from build123d import *

# Parameters (mm, degrees)
BOSS_EXTRUDE1_DEPTH     = 20
SKETCH3_R               = 1.632108338
CUT_EXTRUDE1_DEPTH      = 33.330326321
CUT_EXTRUDE1_DEPTH_BACK = 33.330326321
SKETCH4_W               = 30
SKETCH4_H               = 41
BOSS_EXTRUDE2_DEPTH     = 5
SKETCH6_W               = 25
SKETCH6_H               = 25
BOSS_EXTRUDE3_DEPTH     = 20
CUT_EXTRUDE4_START      = 12.5
CUT_EXTRUDE4_DEPTH      = 20
SKETCH8_W               = 9.9
SKETCH8_H               = 9.9
SKETCH8_W_2             = 15.1
CUT_EXTRUDE5_DEPTH      = 33.330326321
CUT_EXTRUDE5_DEPTH_BACK = 33.330326321


with BuildPart() as part:
    # Sketch2 → Boss-Extrude1 (new body)
    with BuildSketch(Plane.XY):
        Polygon((0, 20.5), (-15, 20.5), (-15, 6.5), (-5.864885696, 6.5), (-5.864885696, -6.5), (-15, -6.5), (-15, -20.5), (0, -20.5), (15, -20.5), (15, -6.5), (5.864885696, -6.5), (5.864885696, 6.5), (15, 6.5), (15, 20.5), align=None)
    extrude(amount=BOSS_EXTRUDE1_DEPTH)

    # Sketch3 → Cut-Extrude1 (cut, two sides)
    with BuildSketch(Plane(origin=(0, 0, 0), x_dir=(1, 0, 0), z_dir=(0, 1, 0))) as cut_extrude1_sk:
        with Locations(Location((-10, -10, 0), (0, 0, 270))):
            Circle(SKETCH3_R)
        with Locations(Location((10, -10, 0), (0, 0, 270))):
            Circle(SKETCH3_R)
    extrude(amount=CUT_EXTRUDE1_DEPTH, mode=Mode.SUBTRACT)
    extrude(cut_extrude1_sk.sketch, amount=-CUT_EXTRUDE1_DEPTH_BACK, mode=Mode.SUBTRACT)

    # Sketch4 → Boss-Extrude2 (add)
    with BuildSketch(Plane.XY):
        Rectangle(SKETCH4_W, SKETCH4_H)
    extrude(amount=BOSS_EXTRUDE2_DEPTH)

    # Sketch6 → Boss-Extrude3 (add)
    with BuildSketch(Plane.XY):
        Rectangle(SKETCH6_W, SKETCH6_H)
    extrude(amount=-BOSS_EXTRUDE3_DEPTH)

    # Sketch7 → Cut-Extrude4 (cut)
    with BuildSketch(Plane(origin=(0, 0, 0), x_dir=(1, 0, 0), z_dir=(0, 1, 0)).offset(CUT_EXTRUDE4_START)):
        Polygon((-2.6, 5.15), (-7.55, 5.15), (-7.55, 0), (0, 0), (0, 10.1), (-2.6, 10.1), align=None)
        Polygon((0, 10.1), (0, 0), (7.55, 0), (7.55, 5.15), (2.6, 5.15), (2.6, 10.1), align=None)
    extrude(amount=-CUT_EXTRUDE4_DEPTH, mode=Mode.SUBTRACT)

    # Sketch8 → Cut-Extrude5 (cut, two sides)
    with BuildSketch(Plane(origin=(0, 0, 0), x_dir=(1, 0, 0), z_dir=(0, 1, 0))) as cut_extrude5_sk:
        with Locations((-7.55, 15.05)):
            Rectangle(SKETCH8_W, SKETCH8_H)
        with Locations((4.95, 15.05)):
            Rectangle(SKETCH8_W_2, SKETCH8_H)
    extrude(amount=CUT_EXTRUDE5_DEPTH, mode=Mode.SUBTRACT)
    extrude(cut_extrude5_sk.sketch, amount=-CUT_EXTRUDE5_DEPTH_BACK, mode=Mode.SUBTRACT)


solid = part.part
Can you work these out from the model? Positions are in its coordinate system, mm. A direction names the side the tool comes from. Coordinates: 2 decimals unless noted, no trailing zeros. Loops run counter-clockwise (first coordinate to the right, second up) from the corner with the lowest first, then second, coordinate; pieces in that order, holes last. Notation, with made-up numbers: (11, 12) - (62, 12) arc R19 cw to (62, 19) - close; hole circle Ø7 at (41, -3). An arc over 180 degrees is marked (long way). Answer as a JSON object with one key per item and string values. Group by question number.
Item 1: If we section it at B-B (x = -10): List the corners of the cut face in (y, z) for me.
Item 2: For pin 1 (5.5 mm diameter, centred on y = 7, z = -6.5, fed in from -X); pin 2 (2.5 mm diameter, centred on x = 9.5, y = -2, fed in from +Z); pin 3 (12 mm diameter, centred on x = 2, z = -6.5, fed in from +Y), each with a flat end and sliding along its axis, tell me the tip position at first contact or that it passes through.
Item 3: If we section it at A-A (z = 10): List the corners of the cut face in (x, y) for me, plus the area to 3 significant figures.
Item 4: If I drill on L1, parallel to X at y = 17, z = 10; L2, parallel to Z at x = -10, y = 10.5; L3, parallel to Z at x = -7.25, y = 3.5, over which ranges is the centre line in solid material (lowest first)? Write a range as from..to.
Item 5: On a 3-axis mill with a long thin cutter (end or side, diameter ignored), from which of +Z, -Z, +X, -X, +Y, -Y can I reach the whole of each face in a straight line? I mean faces 1 (the face through (-2.6, 3, -8)), 2 (the face through (0, -12.5, -5)), 3 (the face through (10, 0, 5)), 4 (the face through (-5, 3, -5.15)). Say none if no direction works.
Item 6: If we section it at D-D (x = -4.5): List the corners of the cut face in (y, z) for me, plus the area to 4 significant figures.
Item 7: If we section it at C-C (y = -13.5): List the corners of the cut face in (x, z) for me.
Item 8: If we mould it in two halves opening along Y, with no side actions, what happens to faces 5 (the face through (-12.5, 0, -5)), 6 (the face through (-9, 12.5, -6)), 7 (the face through (-10, 6.5, 12))? For each: released by +Y, released by -Y, zero draft, split by the parting line, or undercut.
Returned:
{
 "1": {"outline": "(-20.5, 0) - (-12.5, 0) - (-12.5, -10.1) - (12.5, -10.1) - (12.5, 0) - (20.5, 0) - (20.5, 8.37) - (6.5, 8.37) - (6.5, 5) - (-6.5, 5) - (-6.5, 8.37) - (-20.5, 8.37) - close; (-20.5, 11.63) - (-6.5, 11.63) - (-6.5, 20) - (-20.5, 20) - close; (6.5, 11.63) - (20.5, 11.63) - (20.5, 20) - (6.5, 20) - close"},
 "2": {"pin 1": "stops at x = -12.5", "pin 2": "stops at z = 5", "pin 3": "stops at y = 12.5"},
 "3": {"outline": "(-15, -20.5) - (-11.63, -20.5) - (-11.63, -6.5) - (-15, -6.5) - close; (-15, 6.5) - (-11.63, 6.5) - (-11.63, 20.5) - (-15, 20.5) - close; (-8.37, -20.5) - (8.37, -20.5) - (8.37, -6.5) - (5.86, -6.5) - (5.86, 6.5) - (8.37, 6.5) - (8.37, 20.5) - (-8.37, 20.5) - (-8.37, 6.5) - (-5.86, 6.5) - (-5.86, -6.5) - (-8.37, -6.5) - close; (11.63, -20.5) - (15, -20.5) - (15, -6.5) - (11.63, -6.5) - close; (11.63, 6.5) - (15, 6.5) - (15, 20.5) - (11.63, 20.5) - close", "area": "810 mm²"},
 "4": {"L1": "x = -15..-11.63, -8.37..8.37, 11.63..15", "L2": "z = -10.1..8.37, 11.63..20", "L3": "z = -10.1..-5.15, 0..5"},
 "5": {"face 1": "-Z, +Y", "face 2": "-Z, +X, -X, -Y", "face 3": "+Z, +X", "face 4": "+Y"},
 "6": {"outline": "(-20.5, 0) - (-12.5, 0) - (-12.5, -10.1) - (12.5, -10.1) - (12.5, -5.15) - (-7.5, -5.15) - (-7.5, 0) - (20.5, 0) - (20.5, 20) - (-20.5, 20) - close", "area": "969.5 mm²"},
 "7": {"outline": "(-15, 0) - (15, 0) - (15, 20) - (-15, 20) - close; hole circle Ø3.26 at (-10, 10); hole circle Ø3.26 at (10, 10)"},
 "8": {"face 5": "zero draft", "face 6": "released by +Y", "face 7": "undercut"}
}
